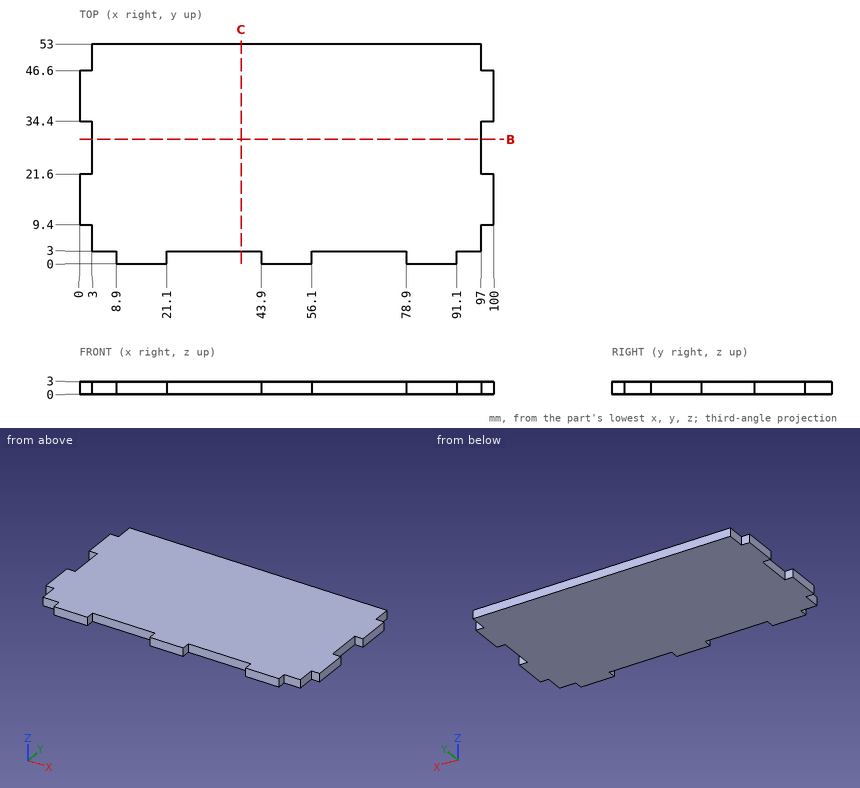
Here's the drawing with two shaded views (mm, measured from the low corner). I have some questions. Round coordinates to 2 decimals unless told otherwise and drop trailing zeros. Write each loop counter-clockwise with the first axis right and the second up, starting at its lowest first coordinate (ties: lowest second). Pieces come first, ordered by that corner, then holes. Notation, with made-up numbers: M -20,-5 L -5,-5 A25 ccw -5,14 Z; hole C 71,-5.5 d2. An arc over 180 degrees is marked long. Answer in a Markdown table with one row per item. Add a question column.
Q1. Imagine slicing it at C-C (x = 39). Please give me the cut outline in (y, z), then the cut area to 3 significant figures.
Q2. Will these pins go through, and if not, where does the flat tip stop? pin 1 Ø0.9 at (y, z) = (1.5, 1) entering from -X; pin 2 Ø1.5 at (x, z) = (2, 1) entering from +Y; pin 3 Ø0.9 at (x, z) = (5.5, 1) entering from -Y.
Q3. Imagine slicing it at B-B (y = 30). Please give me the cut outline in (x, z), then the cut area to 3 significant figures.
Q4. If I drill on line 1 (X direction, y = 6.5, z = 1.4); line 2 (Y direction, x = 61.5, z = 0.5), over which ranges is the centre line in solid material (lowest first)? Write a range as from..to.
Values:
| question | item | result |
|---|---|---|
| 1 | outline | M 3,0 L 53,0 L 53,3 L 3,3 Z |
| 1 | area | 150 mm^2 |
| 2 | pin 1 | x = 8.9 |
| 2 | pin 2 | y = 46.6 |
| 2 | pin 3 | y = 3 |
| 3 | outline | M 3,0 L 97,0 L 97,3 L 3,3 Z |
| 3 | area | 282 mm^2 |
| 4 | line 1 | 3..97 |
| 4 | line 2 | 3..53 |
